Geometry check sheet. Reference: the model listing, model coordinates, mm. Face numbers are marked on the shaded views. A direction names the side the tool comes from. Round coordinates to 2 decimals unless told otherwise and drop trailing zeros. Write each loop counter-clockwise with the first axis right and the second up, starting at its lowest first coordinate (ties: lowest second). Pieces come first, ordered by that corner, then holes. Notation, with made-up numbers: M 38.5,44.25 L 92.5,44.25 A9 ccw 92.5,61.25 Z; hole C 28,24.25 d8. An arc over 180 degrees is marked long. Use a Markdown table: item, result.
```python
from build123d import *

# Parameters (mm, degrees)
SKETCH_1_R      = 3.9
EXTRUDE_1_DEPTH = 0.8
SKETCH_2_R      = 1.5
EXTRUDE_4_DEPTH = 16


with BuildPart() as part:
    # 草图1 → 凸台-拉伸1 (new body)
    with BuildSketch(Plane(origin=(0, 0, 0), x_dir=(1, 0, 0), z_dir=(0, 1, 0))):
        with Locations(Location((0, 0, 0), (0, 0, 270))):
            Circle(SKETCH_1_R)
        Polygon((-1, 0), (-1, 0.2), (-0.2, 0.2), (-0.2, 1), (0, 1), (0.2, 1), (0.2, 0.2), (1, 0.2), (1, 0), (1, -0.2), (0.2, -0.2), (0.2, -1), (0, -1), (-0.2, -1), (-0.2, -0.2), (-1, -0.2), align=None, mode=Mode.SUBTRACT)
    extrude(amount=EXTRUDE_1_DEPTH)

    # 草图2 → 凸台-拉伸4 (add)
    with BuildSketch(Plane(origin=(0, 0.8, 0), x_dir=(1, 0, 0), z_dir=(0, 1, 0))):
        with Locations(Location((0, 0, 0), (0, 0, 270))):
            Circle(SKETCH_2_R)
    extrude(amount=EXTRUDE_4_DEPTH)


solid = part.part
```
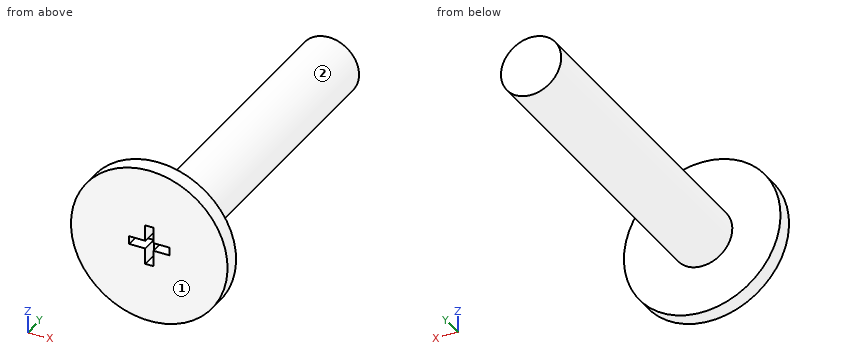
Item 1: Go/stop test with flat-tipped pins: pin 1 (0.6 mm diameter, centred on x = -0.5, y = 0.5, fed in from -Z); pin 2 (0.9 mm diameter, centred on y = 0.5, z = -1, fed in from +X); pin 3 (2 mm diameter, centred on y = 6.5, z = 0.5, fed in from +X). Record where each tip stops, or that it passes through.
Outcome:
| item | result |
|---|---|
| pin 1 | stops at z = -3.89 |
| pin 2 | stops at x = 3.86 |
| pin 3 | stops at x = 1.5 |
Item 2: Cross-section at B-B, the plane z = 0. Record the cut outline in (x, y), and give its area (3 significant figures).
Outcome:
| item | result |
|---|---|
| outline | M -3.9,0 L -1,0 L -1,0.8 L 1,0.8 L 1,0 L 3.9,0 L 3.9,0.8 L 1.5,0.8 L 1.5,16.8 L -1.5,16.8 L -1.5,0.8 L -3.9,0.8 Z |
| area | 52.6 mm2 |
Item 3: Cross-section at A-A, the plane x = 0. Record the cut outline in (y, z), and give its area (3 significant figures).
Outcome:
| item | result |
|---|---|
| outline | M 0,-3.9 L 0.8,-3.9 L 0.8,-1.5 L 16.8,-1.5 L 16.8,1.5 L 0.8,1.5 L 0.8,3.9 L 0,3.9 L 0,1 L 0.8,1 L 0.8,-1 L 0,-1 Z |
| area | 52.6 mm2 |
Item 4: Cross-section at D-D, the plane x = 2.5. Record the cut outline in (y, z), and give its area (3 significant figures).
Outcome:
| item | result |
|---|---|
| outline | M 0,-2.99 L 0.8,-2.99 L 0.8,2.99 L 0,2.99 Z |
| area | 4.79 mm2 |
Item 5: Access from +Z, -Z, +X, -X, +Y, -Y to the whole of each face (thin tool, end or side, straight path). Record for the marked faces 1 and 2.
Outcome:
| item | result |
|---|---|
| face 1 | +Z, -Z, +X, -X, -Y |
| face 2 | +Y |
Item 6: Material ranges on line 1 along Y through (x, z) = (2.5, 1.75); line 2 along Y through (x, z) = (0.75, 0); line 3 along X through (y, z) = (15, -0.25), recorded low to high. Write a range as from..to.
Outcome:
| item | result |
|---|---|
| line 1 | y = 0..0.8 |
| line 2 | y = 0.8..16.8 |
| line 3 | x = -1.48..1.48 |
Item 7: Cross-section at C-C, the plane y = 1. Record the cut outline in (x, z), and give its area (3 significant figures).
Outcome:
| item | result |
|---|---|
| outline | C 0,0 d3 |
| area | 7.07 mm2 |
